from build123d import *

# Parameters (mm, degrees)
CUT_EXTRUDE3_DEPTH           = 60
CUT_EXTRUDE5_DEPTH           = 2
CUT_EXTRUDE5_DEPTH_BACK      = 30
SKETCH19_W                   = 12
SKETCH19_H                   = 36.5
CUT_REVOLVE2_ANGLE           = 65
CUT_REVOLVE2_OTHER_WAY_ANGLE = 65
SKETCH21_W                   = 3.25
SKETCH21_H                   = 4
BOSS_EXTRUDE3_DEPTH          = 1.35
CIRPATTERN1_COUNT            = 5
CUT_EXTRUDE9_START           = -5
CUT_EXTRUDE9_DEPTH           = 5


# Read off the part's stored shape, not the designer's step: Cut-Extrude9
with BuildPart() as part:
    # Sketch1 → Revolve1 (revolve)
    with BuildSketch(Plane.XY, mode=Mode.PRIVATE) as revolve1_sk:
        with BuildLine():
            Line((0, 63.427876097), (32, 63.427876097))
            ThreePointArc((32, 63.427876097), (37.656854249, 61.084730346), (40, 55.427876097))
            Line((40, 55.427876097), (40, 31.556288966))
            ThreePointArc((40, 31.556288966), (38.188122658, 24.409721904), (33.190210564, 18.989648567))
            Line((33.190210564, 18.989648567), (28.539859624, 15.958818353))
            ThreePointArc((28.539859624, 15.958818353), (25.207918228, 12.345436129), (24, 7.581058088))
            Line((24, 7.581058088), (24, 3.25))
            Line((24, 3.25), (24.35, 3))
            Line((24.35, 3), (24.35, 0))
            Line((24.35, 0), (22.5, 0))
            Line((22.5, 0), (22.5, 12.5))
            ThreePointArc((22.5, 12.5), (22.353553391, 12.853553391), (22, 13))
            Line((22, 13), (0, 13))
            Line((0, 13), (0, 63.427876097))
        make_face()
    revolve(revolve1_sk.sketch.rotate(Axis((0, 0, 0), (0, 1, 0)), 90), axis=Axis((0, 0, 0), (0, 1, 0)))

    # Sketch11 → Cut-Extrude3 (cut)
    with BuildSketch(Plane(origin=(0, 13, 0), x_dir=(-1, 0, 0), z_dir=(0, -1, 0))):
        with BuildLine():
            Line((-21, 0), (21, 0))
            ThreePointArc((21, 0), (0, 21), (-21, 0))
        make_face()
    extrude(amount=-CUT_EXTRUDE3_DEPTH, mode=Mode.SUBTRACT)

    # Sketch9 → Cut-Extrude5 (cut, two sides: drawn at the far end of the back side and taken through both)
    with BuildSketch(Plane(origin=(0, 55.427876097, 0), x_dir=(1, 0, 0), z_dir=(0, 1, 0)).offset(-CUT_EXTRUDE5_DEPTH_BACK)):
        with BuildLine():
            ThreePointArc((-37, -1.601545046), (-0.398454954, -39), (37, -2.398454954))
            ThreePointArc((37, -2.398454954), (0.398454954, 35), (-37, -1.601545046))
        make_face()
        with BuildLine():
            Line((-24, -1.763080838), (24, -1.763080838))
            ThreePointArc((24, -1.763080838), (0, 24), (-24, -1.763080838))
        make_face(mode=Mode.SUBTRACT)
    extrude(amount=CUT_EXTRUDE5_DEPTH + CUT_EXTRUDE5_DEPTH_BACK, mode=Mode.SUBTRACT)

    # Sketch19 → Cut-Revolve2 (revolve, cut)
    with BuildSketch(Plane(origin=(0, 0, 0), x_dir=(0, 0, -1), z_dir=(1, 0, 0))):
        with Locations((-41.064715832, 37.177876097)):
            Rectangle(SKETCH19_W, SKETCH19_H)
    revolve(axis=Axis((0, 0, 0), (0, 1, 0)), revolution_arc=CUT_REVOLVE2_ANGLE, mode=Mode.SUBTRACT)

    # Sketch19 → Cut-Revolve2 other way (revolve, cut)
    with BuildSketch(Plane(origin=(0, 0, 0), x_dir=(0, 0, -1), z_dir=(1, 0, 0))):
        with Locations((-41.064715832, 37.177876097)):
            Rectangle(SKETCH19_W, SKETCH19_H)
    revolve(axis=Axis((0, 0, 0), (0, -1, 0)), revolution_arc=CUT_REVOLVE2_OTHER_WAY_ANGLE, mode=Mode.SUBTRACT)

    # Sketch21 → Boss-Extrude3 (add)
    with BuildSketch(Plane(origin=(0, 0, 22.5), x_dir=(-1, 0, 0), z_dir=(0, 0, -1))):
        with Locations((0, 2)):
            Rectangle(SKETCH21_W, SKETCH21_H)
    boss_extrude3 = extrude(amount=BOSS_EXTRUDE3_DEPTH)

    # CirPattern1: Boss-Extrude3 ×5 about axis
    cirpattern1_axis = Axis((0, 0, 0), (0, 1, 0))
    for i in range(1, CIRPATTERN1_COUNT):
        add(boss_extrude3.rotate(cirpattern1_axis, i * 360 / CIRPATTERN1_COUNT))

    # Cut-Extrude9 outline → Cut-Extrude9 (cut)
    with BuildSketch(Plane(origin=(0, 63.427876097, 0), x_dir=(1, 0, 0), z_dir=(0, 1, 0)).offset(CUT_EXTRUDE9_START)):
        with BuildLine():
            ThreePointArc((40, 0), (0, 40), (-40, 0))
            Line((-40, 0), (-21, 0))
            ThreePointArc((-21, 0), (0, 21), (21, 0))
            Line((21, 0), (40, 0))
        make_face()
    extrude(amount=CUT_EXTRUDE9_DEPTH, mode=Mode.SUBTRACT)


solid = part.part
Model file for the job. Use its own axes, mm. A direction names the side the tool comes from. Coordinates: 2 decimals unless noted, no trailing zeros. Write each loop counter-clockwise with the first axis right and the second up, starting at its lowest first coordinate (ties: lowest second). Pieces come first, ordered by that corner, then holes. Notation, with made-up numbers: (-25, 1.5) -> (-12, 1.5) arc R25 cw to (-12, 20.5) -> close; hole circle Ø2 at (61.25, 4). An arc over 180 degrees is marked (long way). One line per item, written item: value. Start each with the question number.
1) Pull direction X, two halves, no side cores. Call faces 1 (the face through (25.5, 16.1, -13.3)), 2 (the face through (12.413, 2.028, -17.124)), 3 (the face through (-12.45, 2.028, -17.097)), 4 (the face through (13, 0, -18)): +X half, -X half, draft (parallel to the pull), parting line (faces both ways), or undercut.
2) Probe probe 1 along Z at (x, y) = (0.5, 42.5); probe 2 along Z at (x, y) = (-2.5, 38.5); probe 3 along Z at (x, y) = (-4.5, 55.5). List the from-to ranges inside material, lowest first.
3) Slice it at D-D on y = 27. Write the cut outline in (x, z), then the cut area to 3 significant figures.
4) Flat gauge pins, fed straight in: pin 1 Ø5 at (y, z) = (16.5, 3.5) entering from -X; pin 2 Ø6 at (x, y) = (10.5, 6.5) entering from -Z; pin 3 Ø6 at (y, z) = (25.5, -23) entering from -X; pin 4 Ø12 at (y, z) = (46, 24) entering from +X. Where does each tip first touch, or does it go through?
5) Which spindle directions (+Z, -Z, +X, -X, +Y, -Y) get a long thin tool onto all of the face, cutting with end or side? Do faces 5 (the face through (0, 35, -21)), 6 (the face through (35.04, 38.18, 16.34)), 7 (the face through (20.122, 2.028, 6.514)), 8 (the face through (-1, 25.428, 7)). Say none if no direction does.
6) Slice it at B-B on x = 0. Count the separate pieces of the cut face and the enclosed holes in it, then the cut area to 3 significant figures.
7) Slice it at A-A on y = 39. Write the cut outline in (x, z).
Answers follow:
1. face 1: parting line
1. face 2: undercut
1. face 3: undercut
1. face 4: draft
2. probe 1: -40 to -35, -23.99 to -20.99, 0 to 1.76
2. probe 2: -39.92 to -34.92, -23.87 to -20.85, 0 to 1.76
2. probe 3: -39.75 to -34.73, -23.58 to -20.51, 0 to 1.76, 38.73 to 39.75
3. outline: (-35.61, 16.61) arc R39.29 ccw (long way) to (35.61, 16.61) -> (34.26, 15.98) arc R37 cw (long way) to (-34.26, 15.98) -> close; (-24, 1.76) arc R24.06 ccw (long way) to (24, 1.76) -> close; hole (-21, 0) arc R21 ccw to (21, 0) -> close
3. area: 785 mm2
4. pin 1: x = -33.03
4. pin 2: z = -22.8
4. pin 3: x = -33.58
4. pin 4: through
5. face 5: +Y, -Y
5. face 6: +Z, -Y
5. face 7: -Y
5. face 8: none
6. separate pieces: 2
6. enclosed holes: 1
6. area: 1,150 mm2
7. outline: (-36.25, 16.9) arc R40 ccw (long way) to (36.25, 16.9) -> (34.26, 15.98) arc R37 cw (long way) to (-34.26, 15.98) -> close; (-24, 1.76) arc R24.06 ccw (long way) to (24, 1.76) -> close; hole (-21, 0) arc R21 ccw to (21, 0) -> close
